Source: CAD feature listing. Evaluate the final solid. Frame: model axes, mm. A direction names the side the tool comes from. Give positions to 0.01 mm unless a question says otherwise; leave off trailing zeros. Order: outer loops, then holes, each group sorted by start corner. A loop starts at its lowest first (then second) coordinate and runs counter-clockwise, first axis right, second up.
Autodesk Inventor part; units mm, degrees
ref_plane "YZ Plane" through (0, 0, 0) normal (1, 0, 0) x (0, 1, 0)
ref_plane "XZ Plane" through (0, 0, 0) normal (0, 1, 0) x (-1, 0, 0)
ref_plane "XY Plane" through (0, 0, 0) normal (0, 0, 1) x (1, 0, 0)
sketch "Sketch1" plane through (0, 0, 0) normal (0, 0, 1) x (1, 0, 0)
  line L0 (0, 0) -> (35, 0)
  line L1 (45, 10) -> (45, 200)
  line L2 (0, 200) -> (0, 0)
  arc A0 (35, 0) -> (45, 10) centre (35, 10) ccw
  line L3 (41.5, 200) -> (41.5, 10)
  arc A1 (35, 3.5) -> (41.5, 10) centre (35, 10) ccw
  line L4 (35, 3.5) -> (0, 3.5)
  line L5 (41.5, 200) -> (45, 200)
  line L6 (0, 3.5) -> (0, 0)
  point P0 (45, 0)
  dimension "d0" = 90
  dimension "d1" = 200
  dimension "d2" = 10
  dimension "d5" = 3.5
  dimension "d6" = 3.5
revolve "Revolution1" add sketch "Sketch1" angle 360 about axis through (0, 200, 0) along (0, -1, 0)
sketch "Sketch2" plane through (0, 200, 0) normal (0, 1, 0) x (1, 0, 0)
  circle A0 centre (0, 0) radius 45 construction
  line L0 (0, 45) -> (0, -45) construction
  line L1 (-45, 0) -> (45, 0) construction
  circle A1 centre (0, 0) radius 45 construction
  circle A2 centre (0, 0) radius 41.5 construction
  circle A3 centre (0, 0) radius 41.5 construction
  circle A4 centre (0, 0) radius 45 construction
  line L2 (0, -41.5) -> (0, -45) construction
  line L3 (-2.5, -45.45) -> (2.5, -45.45)
  line L4 (2.5, -45.45) -> (2.5, -41.05)
  line L5 (2.5, -41.05) -> (-2.5, -41.05)
  line L6 (-2.5, -41.05) -> (-2.5, -45.45)
  line L7 (-2.5, -45.45) -> (2.5, -41.05) construction
  line L8 (2.5, -45.45) -> (-2.5, -41.05) construction
  point P0 (0, -43.25)
  dimension "d8" = 5
  dimension "d9" = 4.4
extrude "Extrusion1" cut sketch "Sketch2" against normal blind 180
fillet "Fillet1" radius 1 2 edges at (-2.5, 200, 43.1776) (2.5, 200, 43.1776)
sketch "Sketch3" plane through (0, 200, 0) normal (0, 1, 0) x (1, 0, 0)
  arc A0 (3.5, -41.3521) -> (-3.5, -41.3521) centre (0, 0) ccw
  circle A1 centre (0, 0) radius 42.5
  circle A2 centre (0, 0) radius 41.5
  point P0 (3.5, -41.3521)
  point P1 (-3.5, -41.3521)
  dimension "d13" = 85
extrude "Extrusion2" cut sketch "Sketch3" against normal blind 5
properties part number "Exterior" material "ABS Plastic"
1) Material intervals for L1, parallel to X at y = 97, z = -1; L2, parallel to X at y = 196, z = 0; L3, parallel to Z at x = 0, y = 80, sorted ascending.
Report:
L1: x = -44.99 to -41.49, 41.49 to 44.99
L2: x = -45 to -42.5, 42.5 to 45
L3: z = -45 to -41.5
2) Section query B-B, the plane z = 0. Return the cut outline in (x, y), and give its area (3 significant figures).
Report:
outline: (-45, 10) arc R10 ccw to (-35, 0) - (35, 0) arc R10 ccw to (45, 10) - (45, 200) - (42.5, 200) - (42.5, 195) - (41.5, 195) - (41.5, 10) arc R6.5 cw to (35, 3.5) - (-35, 3.5) arc R6.5 cw to (-41.5, 10) - (-41.5, 195) - (-42.5, 195) - (-42.5, 200) - (-45, 200) - close
area: 1,660 mm2
3) Section query A-A, the plane x = 0. Return the cut outline in (y, z).
Report:
outline: (0, -35) arc R10 ccw to (10, -45) - (200, -45) - (200, -42.5) - (195, -42.5) - (195, -41.5) - (10, -41.5) arc R6.5 cw to (3.5, -35) - (3.5, 35) arc R6.5 cw to (10, 41.5) - (20, 41.5) - (20, 45) - (10, 45) arc R10 ccw to (0, 35) - close
4) Draft query along Z for faces 1 (the flat face through (0, 0, 0)), 2 (the cylindrical face through (1.83, 197.54, -42.46)), 3 (the cylindrical face through (20.765, 106.33, 39.923)). Return one class per face: +Z half, -Z half, draft (parallel to the pull), parting line (faces both ways), or undercut.
Report:
face 1: draft
face 2: undercut
face 3: parting line
5) Reachability of faces 4 (the flat face through (-26.9, 200, -33.1)), 5 (the cylindrical face through (39.584, 101.205, 12.465)), 6 (the flat face through (0, 20, 43)) from +Z, -Z, +X, -X, +Y, -Y: full face, straight path, thin tool, end or side. Return the list, or none.
Report:
face 4: +Z, -Z, +X, -X, +Y
face 5: +Y
face 6: +Z, +Y
6) Pin query (flat end, axial travel): pin 1 (12 mm diameter, centred on y = 99.5, z = 16, fed in from +X); pin 2 (4 mm diameter, centred on y = 91, z = 42.5, fed in from +X); pin 3 (4 mm diameter, centred on y = 53, z = -15.5, fed in from -X). Return the tip coordinate at first contact, or that it passes through.
Report:
pin 1: stops at x = 43.87
pin 2: stops at x = 19.62
pin 3: stops at x = -42.93
7) Section query C-C, the plane y = 131. Return the cut outline in (x, z), and give its area (3 significant figures).
Report:
outline: (-2.5, 41.42) - (-2.5, 44.93) arc R45 ccw (long way) to (2.5, 44.93) - (2.5, 41.42) arc R41.5 cw (long way) to start
area: 934 mm2
